```python
from build123d import *

# Parameters (mm, degrees)
MAINBODY_DEPTH      = 5
BOSS_EXTRUDE4_DEPTH = 10
FILLET4_R           = 1.27


with BuildPart() as part:
    # Sketch1 → MainBody (new, symmetric)
    with BuildSketch(Plane(origin=(0, 0, 0), x_dir=(0, 0, -1), z_dir=(1, 0, 0))):
        Polygon((106.918290099, 0.604217668), (93.456290099, 0.604217668), (93.456290099, -10.825782332), (106.918290099, -10.825782332), (106.918290099, -7.460282332), (104.886290099, -7.460282332), (104.886290099, -8.476282332), (95.424790099, -8.476282332), (95.424790099, -1.745282332), (104.886290099, -1.745282332), (104.886290099, -2.761282332), (106.918290099, -2.761282332), align=None)
    extrude(amount=MAINBODY_DEPTH, both=True)

    # Sketch10 → Boss-Extrude4 (add)
    with BuildSketch(Plane(origin=(5, 0, 0), x_dir=(0, 0, -1), z_dir=(1, 0, 0))):
        with BuildLine():
            Line((91.170290099, -5.809282332), (91.170290099, -5.110782332))
            Line((91.170290099, -5.110782332), (91.170290099, -4.412282332))
            Line((91.170290099, -4.412282332), (92.380127588, -4.412282332))
            ThreePointArc((92.380127588, -4.412282332), (89.773290099, -5.110782332), (92.380127588, -5.809282332))
            Line((92.380127588, -5.809282332), (91.170290099, -5.809282332))
        make_face()
        with BuildLine():
            Line((91.170290099, -4.412282332), (91.170290099, -5.110782332))
            Line((91.170290099, -5.110782332), (92.567290099, -5.110782332))
            ThreePointArc((92.567290099, -5.110782332), (92.519688478, -4.749212126), (92.380127588, -4.412282332))
            Line((92.380127588, -4.412282332), (91.170290099, -4.412282332))
        make_face()
        with BuildLine():
            Line((92.567290099, -5.110782332), (91.170290099, -5.110782332))
            Line((91.170290099, -5.110782332), (91.170290099, -5.809282332))
            Line((91.170290099, -5.809282332), (92.380127588, -5.809282332))
            ThreePointArc((92.380127588, -5.809282332), (92.519688478, -5.472352538), (92.567290099, -5.110782332))
        make_face()
        with BuildLine():
            ThreePointArc((92.380127588, -4.412282332), (92.519688478, -4.749212126), (92.567290099, -5.110782332))
            Line((92.567290099, -5.110782332), (93.456290099, -5.110782332))
            Line((93.456290099, -5.110782332), (93.456290099, -4.412282332))
            Line((93.456290099, -4.412282332), (92.380127588, -4.412282332))
        make_face()
        with BuildLine():
            Line((93.456290099, -5.110782332), (92.567290099, -5.110782332))
            ThreePointArc((92.567290099, -5.110782332), (92.519688478, -5.472352538), (92.380127588, -5.809282332))
            Line((92.380127588, -5.809282332), (93.456290099, -5.809282332))
            Line((93.456290099, -5.809282332), (93.456290099, -5.110782332))
        make_face()
    extrude(amount=-BOSS_EXTRUDE4_DEPTH)

    # Fillet4
    fillet4_edges = [part.edges().sort_by_distance(p)[0] for p in [
        (0, -1.745282332, -95.424790099),
        (0, -8.476282332, -95.424790099),
        (0, -10.825782332, -106.918290099),
        (0, -10.825782332, -93.456290099),
        (0, 0.604217668, -93.456290099),
        (0, 0.604217668, -106.918290099),
    ]]
    fillet(fillet4_edges, radius=FILLET4_R)


solid = part.part
```
Check sheet for the modelled part. Datum: model origin and axes. Units: mm. A direction names the side the tool comes from. Round coordinates to 2 decimals unless told otherwise and drop trailing zeros. Order: outer loops, then holes, each group sorted by start corner. A loop starts at its lowest first (then second) coordinate and runs counter-clockwise, first axis right, second up.
1) Go/stop test with flat-tipped pins: pin 1 Ø1.1 at (x, y) = (-2, -8) entering from +Z; pin 2 Ø0.5 at (x, z) = (-1.5, -93) entering from -Y; pin 3 Ø2 at (x, z) = (2.5, -93.5) entering from -Y. Record where each tip stops, or that it passes through.
2) Mould release check, pull along Z, two halves, no side actions. Record for faces 1 (the flat face through (0, 0.604, -100)), 2 (the cylindrical face through (0.07, -2.127, -95.787)), 3 (the cylindrical face through (0.07, 0.242, -93.838)), 4 (the flat face through (0, -5, -95.425)): +Z half, -Z half, draft (parallel to the pull), parting line (faces both ways), or undercut.
3) Section check C-C (x = 3.25). Record the boundary of the cut face in (y, z).
4) Section check B-B (y = -2.25). Record the boundary of the cut face in (x, z).
5) Section check D-D (y = -1). Record the boundary of the cut face in (x, z), and give its area (3 significant figures).
6) Scan lines: line 1 (Y direction, x = -1.5, z = -104.5); line 2 (Z direction, x = 2.75, y = -9.25); line 3 (Z direction, x = 0, y = -5). Record each from-to range of solid material in increasing order.
7) Tool access check on faces 5 (the flat face through (0, -2, -104.886)), 6 (the flat face through (0, -4.412, -93)), 7 (the flat face through (0, -8, -93.456)). Record the directions out of +Z, -Z, +X, -X, +Y, -Y that give a thin tool (end or side, any length) a straight path to the whole face; none if there is none.
8) Section check A-A (z = -99.5). Record the boundary of the cut face in (x, y), and give its area (3 significant figures).
Result:
1. pin 1: stops at z = -93.46
1. pin 2: stops at y = -5.81
1. pin 3: stops at y = -10.81
2. face 1: draft
2. face 2: undercut
2. face 3: +Z half
2. face 4: -Z half
3. outline: (-10.83, -105.65) arc R1.27 ccw to (-9.56, -106.92) - (-7.46, -106.92) - (-7.46, -104.89) - (-8.48, -104.89) - (-8.48, -96.69) arc R1.27 cw to (-7.21, -95.42) - (-3.02, -95.42) arc R1.27 cw to (-1.75, -96.69) - (-1.75, -104.89) - (-2.76, -104.89) - (-2.76, -106.92) - (-0.67, -106.92) arc R1.27 ccw to (0.6, -105.65) - (0.6, -94.73) arc R1.27 ccw to (-0.67, -93.46) - (-4.41, -93.46) - (-4.41, -92.38) arc R1.4 ccw (long way) to (-5.81, -92.38) - (-5.81, -93.46) - (-9.56, -93.46) arc R1.27 ccw to (-10.83, -94.73) - close
4. outline: (-5, -106.92) - (5, -106.92) - (5, -104.89) - (-5, -104.89) - close; (-5, -95.68) - (5, -95.68) - (5, -93.46) - (-5, -93.46) - close
5. outline: (-5, -106.92) - (5, -106.92) - (5, -93.46) - (-5, -93.46) - close
5. area: 135 mm2
6. line 1: y = -10.83 to -8.48, -1.75 to 0.6
6. line 2: z = -106.92 to -93.46
6. line 3: z = -95.42 to -89.78
7. face 5: +X, -X
7. face 6: +X, -X, +Y
7. face 7: +X, -X, -Y
8. outline: (-5, -10.83) - (5, -10.83) - (5, -8.48) - (-5, -8.48) - close; (-5, -1.75) - (5, -1.75) - (5, 0.6) - (-5, 0.6) - close
8. area: 47.0 mm2
